Geometry: final body of the model. Coordinates: model frame, mm. A direction names the side the tool comes from. Round coordinates to 2 decimals unless told otherwise and drop trailing zeros. Loops run counter-clockwise (first coordinate to the right, second up) from the corner with the lowest first, then second, coordinate; pieces in that order, holes last. Notation, with made-up numbers: M 47,-1 L 100,-1 A23 ccw 100,30 Z; hole C 2.5,-11 d7. An arc over 180 degrees is marked long. Write each question's results on one line, items separated by ' | '.
```python
from build123d import *

# Parameters (mm, degrees)
ESBO_O1_W                 = 105
ESBO_O1_H                 = 60
RESSALTO_EXTRUS_O1_DEPTH  = 1.7
RESSALTO_EXTRUS_O6_START  = 11.6
ESBO_O3_W                 = 100
ESBO_O3_H                 = 53
RESSALTO_EXTRUS_O6_DEPTH  = 1.5
ESBO_O4_W                 = 62.184169383
ESBO_O4_H                 = 2.54
ESBO_O4_W_2               = 5.08
ESBO_O4_H_2               = 42.957805244
ESBO_O4_W_3               = 56.07185462
RESSALTO_EXTRUS_O8_DEPTH  = 11.6
ESBO_O7_W                 = 25.746964405
ESBO_O7_H                 = 12
RESSALTO_EXTRUS_O10_DEPTH = 10
ESBO_O8_R                 = 1.5
ESBO_O8_W                 = 105
ESBO_O8_H                 = 7.9
CORTE_EXTRUS_O1_DEPTH     = 15.8
ESBO_O9_W                 = 120.671020404
ESBO_O9_H                 = 64.953228707
RESSALTO_EXTRUS_O11_DEPTH = 1.7


with BuildPart() as part:
    # Esbo_o1 → Ressalto-extrus_o1 (new body)
    with BuildSketch(Plane.XY):
        Rectangle(ESBO_O1_W, ESBO_O1_H)
    extrude(amount=RESSALTO_EXTRUS_O1_DEPTH)



with BuildPart() as body_2:
    # Esbo_o3 → Ressalto-extrus_o6 (new body)
    with BuildSketch(Plane(origin=(0, 0, 0), x_dir=(-1, 0, 0), z_dir=(0, 0, -1)).offset(RESSALTO_EXTRUS_O6_START)):
        with Locations((2.5, 4.4)):
            Rectangle(ESBO_O3_W, ESBO_O3_H)
    extrude(amount=RESSALTO_EXTRUS_O6_DEPTH)


with BuildPart() as part_1:
    add(part.part)

    add(body_2.part)  # Ressalto-extrus_o8 merges body 2
    # Esbo_o4 → Ressalto-extrus_o8 (add)
    with BuildSketch(Plane.XY.offset(-11.6)):
        with Locations((7.150543675, 26.719832293)):
            Rectangle(ESBO_O4_W, ESBO_O4_H)
        with Locations((45.784919315, 5.42627648)):
            Rectangle(ESBO_O4_W_2, ESBO_O4_H_2)
        with Locations((10.206701056, -18.689881399)):
            Rectangle(ESBO_O4_W_3, ESBO_O4_H)
    extrude(amount=RESSALTO_EXTRUS_O8_DEPTH)

    # Esbo_o7 → Ressalto-extrus_o10 (add)
    with BuildSketch(Plane.XY.offset(-11.6)):
        with Locations((-47.626517798, 17.9)):
            Rectangle(ESBO_O7_W, ESBO_O7_H)
    extrude(amount=RESSALTO_EXTRUS_O10_DEPTH)

    # Esbo_o8 → Corte-extrus_o1 (cut, through all)
    with BuildSketch(Plane(origin=(0, 0, -13.1), x_dir=(-1, 0, 0), z_dir=(0, 0, -1))):
        with Locations((37.26, 28.47)):
            Circle(ESBO_O8_R)
        with Locations((38.5, -19.7)):
            Circle(ESBO_O8_R)
        with Locations((-43.8, -19.7)):
            Circle(ESBO_O8_R)
        with Locations((0, -26.05)):
            Rectangle(ESBO_O8_W, ESBO_O8_H)
    extrude(amount=-CORTE_EXTRUS_O1_DEPTH, mode=Mode.SUBTRACT)

    # Esbo_o9 → Ressalto-extrus_o11 (add)
    with BuildSketch(Plane.XY.offset(1.7)):
        with Locations((2.076306878, 11.29693703)):
            Rectangle(ESBO_O9_W, ESBO_O9_H)
    extrude(amount=-RESSALTO_EXTRUS_O11_DEPTH)


solid = part_1.part
```
1. Ray query, probe 1 along X at (y, z) = (17.5, -10); probe 2 along Z at (x, y) = (10.5, -9.5); probe 3 along Y at (x, z) = (-37.26, -12.8). Return the intervals inside material, ascending.
Answer key:
probe 1: x = -60.5 to -34.75, 43.24 to 48.32 | probe 2: z = -13.1 to -11.6, 0 to 1.7 | probe 3: y = -22.1 to -20.54, -18.86 to 26.97, 29.97 to 30.9
2. Section B-B (z = -6). Output: boundary loops of the cut face in (x, y), then the cut area to 3 significant figures.
Answer key:
outline: M -60.5,11.9 L -34.75,11.9 L -34.75,23.9 L -60.5,23.9 Z; M -23.94,25.45 L 38.24,25.45 L 38.24,27.99 L -23.94,27.99 Z; M -17.83,-19.96 L 38.24,-19.96 L 38.24,-17.42 L -17.83,-17.42 Z; M 43.24,-16.05 L 48.32,-16.05 L 48.32,26.91 L 43.24,26.91 Z | area: 828 mm²
3. Draft query along Z for faces 1 (the face through (-38.69, 28.92, -12.36)), 2 (the face through (-48, 11.9, -7)), 3 (the face through (-2, 5, -13.1)). Return one class per face: pulls with the +Z half, pulls with the -Z half, needs draft (parallel to the pull), parting line crosses it, or undercut.
Answer key:
face 1: needs draft | face 2: undercut | face 3: pulls with the -Z half
4. Section D-D (y = -4). Output: boundary loops of the cut face in (x, z), then the cut area to 3 significant figures.
Answer key:
outline: M -58.26,0 L 43.24,0 L 43.24,-11.6 L -52.5,-11.6 L -52.5,-13.1 L 47.5,-13.1 L 47.5,-11.6 L 48.32,-11.6 L 48.32,0 L 62.41,0 L 62.41,1.7 L -58.26,1.7 Z | area: 414 mm²
5. Section A-A (x = -2.5). Output: boundary loops of the cut face in (y, z).
Answer key:
outline: M -22.1,-13.1 L 30.9,-13.1 L 30.9,-11.6 L 27.99,-11.6 L 27.99,0 L 43.77,0 L 43.77,1.7 L -22.1,1.7 L -22.1,0 L -19.96,0 L -19.96,-11.6 L -22.1,-11.6 Z; hole M -17.42,-11.6 L 25.45,-11.6 L 25.45,0 L -17.42,0 Z
6. Access query for faces 4 (the face through (10, -19.96, -6)), 5 (the face through (43.245, 5, -6)), 6 (the face through (38.243, -19, -6)). Directions: +Z, -Z, +X, -X, +Y, -Y. A direction counts if a zero-diameter tool reaches every point of the face in a straight line with its end or side. Return the directions, or none.
Answer key:
face 4: +X, -X, -Y | face 5: +Y, -Y | face 6: +X, +Y, -Y
7. Pin query (flat end, axial travel): P1, Ø1.3, axis at y = -18.5, z = -4.5, coming from the +X side; P2, Ø1.2, axis at y = 8, z = -12, coming from the +X side; P3, Ø5, axis at x = -48.5, z = -7.5, coming from the +Y side. Return the tip coordinate at first contact, or that it passes through.
Answer key:
P1: stops at x = 38.24 | P2: stops at x = 48.32 | P3: stops at y = 23.9
8. Section C-C (x = -44.5). Output: boundary loops of the cut face in (y, z).
Answer key:
outline: M -22.1,-13.1 L 30.9,-13.1 L 30.9,-11.6 L 23.9,-11.6 L 23.9,-1.6 L 11.9,-1.6 L 11.9,-11.6 L -22.1,-11.6 Z; M -22.1,0 L 43.77,0 L 43.77,1.7 L -22.1,1.7 Z
